Build history of the part. All positions in model axes, mm. A direction names the side the tool comes from. Round coordinates to 2 decimals unless told otherwise and drop trailing zeros. Write each loop counter-clockwise with the first axis right and the second up, starting at its lowest first coordinate (ties: lowest second). Pieces come first, ordered by that corner, then holes.
1) Wall check: probe 1 along Z at (x, y) = (1.75, -13); probe 2 along Z at (x, y) = (3.6, -15); probe 3 along Y at (x, z) = (3.6, 14). Give the ranges that are in metal, low to high.
2) Pull direction Y, two halves, no side cores. Call faces 6 (the flat face through (2, 8.5, -82)), 7 (the flat face through (2, -11, -84)), 8 (the flat face through (2, -13.5, 82)): +Y half, -Y half, draft (parallel to the pull), parting line (faces both ways), or undercut.
3) Which spindle directions (+Z, -Z, +X, -X, +Y, -Y) get a long thin tool onto all of the face, cutting with end or side? Do faces 1 (the flat face through (0, 0, 1)), 2 (the flat face through (2, -8.5, -82)), 3 (the flat face through (2, -15, 60)), 4 (the flat face through (2, 15, 80)), 5 (the flat face through (2, -1.65, 78)). Say none if no direction does.
4) Saw through at A-A (z = 19). Write the cut outline in (x, y).
5) Flat gauge pin, fed straight in: pin 1 (0.9 mm diameter, centred on x = 2, y = -14.5, fed in from +Z). Where does the tip first touch, or does it go through?
6) Saw through at B-B (x = 1.2). State how many separate pieces and enclosed holes the cut face has, plus the area to 3 significant figures.
from build123d import *

# Parameters (mm, degrees)
F0_W     = 4
F0_H     = 20
F1_DEPTH = 4
F2_R     = 2


with BuildPart() as f1:
    # F0 (on Right) → F1 (new body)
    with BuildSketch(Plane.YZ):
        Polygon((13.5, -80), (18.5, -80), (18.5, 80), (13.5, 80), (13.5, 84), (8.5, 84), (8.5, 80), (1.65, 80), (1.65, 76.5), (2.8, 76.5), (2.8, 74), (1.65, 74), (1.65, 72), (-1.65, 72), (-1.65, 74), (-2.8, 74), (-2.8, 76.5), (-1.65, 76.5), (-1.65, 80), (-8.5, 80), (-8.5, 84), (-13.5, 84), (-13.5, 80), (-18.5, 80), (-18.5, -80), (-13.5, -80), (-13.5, -84), (-8.5, -84), (-8.5, -80), (-1.65, -80), (-1.65, -76.5), (-2.8, -76.5), (-2.8, -74), (-1.65, -74), (-1.65, -72), (1.65, -72), (1.65, -74), (2.8, -74), (2.8, -76.5), (1.65, -76.5), (1.65, -80), (8.5, -80), (8.5, -84), (13.5, -84), align=None)
        with Locations((-14.5, -50)):
            Rectangle(F0_W, F0_H, mode=Mode.SUBTRACT)
        Polygon((-8.257359, -56.071068), (-6.843146, -54.656854), (-5.428932, -53.242641), (0.227922, -58.899495), (-1.186292, -60.313708), (-2.600505, -61.727922), align=None, mode=Mode.SUBTRACT)
        Polygon((14.257359, -72.928932), (12.843146, -74.343146), (11.428932, -75.757359), (5.772078, -70.100505), (7.186292, -68.686292), (8.600505, -67.272078), align=None, mode=Mode.SUBTRACT)
        with Locations((14.5, -20)):
            Rectangle(F0_W, F0_H, mode=Mode.SUBTRACT)
        Polygon((-16.5, -10), (-16.5, 0), (-16.5, 10), (-12.5, 10), (-12.5, 0), (-12.5, -10), align=None, mode=Mode.SUBTRACT)
        with Locations((-14.5, 50)):
            Rectangle(F0_W, F0_H, mode=Mode.SUBTRACT)
        Polygon((12.5, 10), (12.5, 20), (12.5, 30), (16.5, 30), (16.5, 20), (16.5, 10), align=None, mode=Mode.SUBTRACT)
        with Locations((14.5, 60)):
            Rectangle(F0_W, F0_H, mode=Mode.SUBTRACT)
    extrude(amount=F1_DEPTH)

    # F2
    f2_edges = [f1.edges().sort_by_distance(p)[0] for p in [
        (2, -18.5, -80),
        (2, 18.5, -80),
        (2, -18.5, 80),
        (2, 18.5, 80),
    ]]
    fillet(f2_edges, radius=F2_R)


solid = f1.part
Evaluation:
1. probe 1: z = -84 to -60, -40 to -10, 10 to 40, 60 to 84
1. probe 2: z = -80 to -60, -40 to -10, 10 to 40, 60 to 80
1. probe 3: y = -18.5 to 12.5, 16.5 to 18.5
2. face 6: undercut
2. face 7: draft
2. face 8: -Y half
3. face 1: +Z, -Z, -X, +Y, -Y
3. face 2: -Z, +X, -X
3. face 3: +X, -X
3. face 4: +Z, +X, -X, +Y
3. face 5: +Z, +X, -X
4. outline: (0, -18.5) - (4, -18.5) - (4, 12.5) - (0, 12.5) - close; (0, 16.5) - (4, 16.5) - (4, 18.5) - (0, 18.5) - close
5. pin 1: stops at z = 80
6. separate pieces: 1
6. enclosed holes: 8
6. area: 5,390 mm2
